Verification items for the finished model (mm, model axes). Face numbers are marked on the shaded views. A direction names the side the tool comes from. Coordinates: 2 decimals unless noted, no trailing zeros. Loops run counter-clockwise (first coordinate to the right, second up) from the corner with the lowest first, then second, coordinate; pieces in that order, holes last. Notation, with made-up numbers: (37, 32) -> (79, 32) arc R35 ccw to (79, 70) -> close; hole circle Ø3 at (27, 32). An arc over 180 degrees is marked (long way). Answer as a JSON object with one key per item and string values. Group by question number.
Q1. Gauge pin test, flat ends, axial feed: pin 1 Ø1.5 at (x, y) = (-14.5, 18) entering from -Z; pin 2 Ø5.5 at (y, z) = (-1.5, 57) entering from +X; pin 3 Ø0.9 at (x, z) = (10.5, 58) entering from +Y; pin 4 Ø2.5 at (x, z) = (10.5, 58) entering from -Y. Record the tip position at first contact, or that the pin passes through.
Q2. Cross-section at A-A on y = -1.5. Record the boundary of the cut face in (x, z), and give its area (3 significant figures).
Q3. Release check for a two-part mould opening along X. For the marked faces 1, 2 and 3 record: released by +X, released by -X, zero draft, split by the parting line, or undercut.
Q4. Cross-section at B-B on x = -23.5. Record the boundary of the cut face in (y, z).
Q5. Scan lines: L1, parallel to Y at x = 7.5, z = 44; L2, parallel to X at y = -16, z = 7; L3, parallel to Z at x = 4.5, y = 4. Record each from-to range of solid material in increasing order.
Q6. Cross-section at C-C on z = 33.5. Record the boundary of the cut face in (x, y), and give its area (3 significant figures).
Q7. Set-up check for the marked faces 4 and 5: record each of +Z, -Z, +X, -X, +Y, -Y from which the full face is reachable in a straight line by a thin tool's end or side.
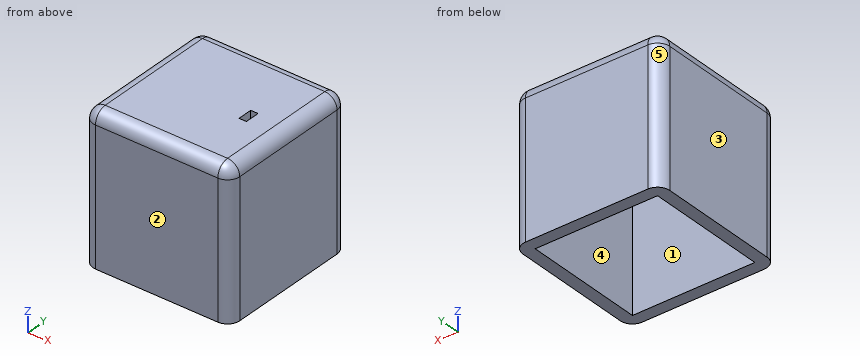
```python
from build123d import *

# Parameters (mm, degrees)
F0_W     = 60
F0_H     = 60
F1_DEPTH = 60
F2_R     = 5
F3_T     = 5
F4_W     = 3
F4_H     = 6
F5_DEPTH = 25


# Not quite as in the source:
# - a shell that OpenCascade refuses in one call is made with other operations: the cavity is built on its own and cut out


with BuildPart() as f1:
    # F0 (on Top) → F1 (new body)
    with BuildSketch(Plane.XY):
        with Locations((-4.3964601223, -1.0684304871)):
            Rectangle(F0_W, F0_H)
    extrude(amount=F1_DEPTH)

    # F2
    f2_edges = [f1.edges().sort_by_distance(p)[0] for p in [
        (25.60354, 28.93157, 30),
        (-4.39646, 28.93157, 60),
        (-34.39646, 28.93157, 30),
        (-34.39646, -1.06843, 60),
        (-34.39646, -31.06843, 30),
        (-4.39646, -31.06843, 60),
        (25.60354, -31.06843, 30),
        (25.60354, -1.06843, 60),
    ]]
    fillet(f2_edges, radius=F2_R)

    # F3: shell of thickness 5, made by hand


with BuildPart() as f3_core1:
    # F3_t2: copy of F1
    add(f1.part)

    # the walls: a layer under each face that stays
    f3_faces = [f3_core1.faces().sort_by_distance(p)[0] for p in [
        (-4.3964601223, 28.9315695129, 27.5),
        (25.6035398777, -1.0684304871, 27.5),
        (-34.3964601223, -1.0684304871, 27.5),
        (-4.3964601223, -31.0684304871, 27.5),
        (-4.3964601223, -1.0684304871, 60),
    ]]
    thicken(f3_faces, amount=-F3_T, mode=Mode.SUBTRACT)


with BuildPart() as f1_1:
    add(f1.part)

    # what is left inside the walls is the cavity
    f3_cavity = [f3_core1.part.solids().sort_by_distance(p)[0] for p in [
        (20.55354, -1.06843, 36.666667),
    ]]
    add(f3_cavity, mode=Mode.SUBTRACT)

    # F4 (on face) → F5 (cut)
    with BuildSketch(Plane.XY.offset(60)):
        with Locations((10.4050671086, -2.4284604266)):
            Rectangle(F4_W, F4_H)
    extrude(amount=-F5_DEPTH, mode=Mode.SUBTRACT)


solid = f1_1.part
```
Computed values:
{
 "1": {"pin 1": "stops at z = 55", "pin 2": "stops at x = 25.6", "pin 3": "stops at y = 28.23", "pin 4": "stops at y = -30.75"},
 "2": {"outline": "(-34.4, 0) -> (-29.4, 0) -> (-29.4, 55) -> (8.91, 55) -> (8.91, 60) -> (-29.4, 60) arc R5 ccw to (-34.4, 55) -> close; (11.91, 55) -> (20.6, 55) -> (20.6, 0) -> (25.6, 0) -> (25.6, 55) arc R5 ccw to (20.6, 60) -> (11.91, 60) -> close", "area": "824 mm²"},
 "3": {"face 1": "undercut", "face 2": "zero draft", "face 3": "released by -X"},
 "4": {"outline": "(-31.07, 0) -> (-26.07, 0) -> (-26.07, 55) -> (23.93, 55) -> (23.93, 0) -> (28.93, 0) -> (28.93, 55) arc R5 ccw to (23.93, 60) -> (-26.07, 60) arc R5 ccw to (-31.07, 55) -> close"},
 "5": {"L1": "y = -31.07 to -26.07, 23.93 to 28.93", "L2": "x = -34.4 to -29.4, 20.6 to 25.6", "L3": "z = 55 to 60"},
 "6": {"outline": "(-34.4, -26.07) arc R5 ccw to (-29.4, -31.07) -> (20.6, -31.07) arc R5 ccw to (25.6, -26.07) -> (25.6, 23.93) arc R5 ccw to (20.6, 28.93) -> (-29.4, 28.93) arc R5 ccw to (-34.4, 23.93) -> close; hole (-29.4, -26.07) -> (20.6, -26.07) -> (20.6, 23.93) -> (-29.4, 23.93) -> close", "area": "1,080 mm²"},
 "7": {"face 4": "-Z", "face 5": "+Z, -Z, -X, +Y"}
}
